Could you check a few things on this model? Use its own coordinates, in mm. A direction names the side the tool comes from. Round coordinates to 2 decimals unless told otherwise and drop trailing zeros. Order: outer loops, then holes, each group sorted by start corner. A loop starts at its lowest first (then second) coordinate and runs counter-clockwise, first axis right, second up.
```python
from build123d import *

# Parameters (mm, degrees)
EXTRUDE_1_DEPTH        = 60
HOLE_WIZARD_M6_1_D     = 5
HOLE_WIZARD_M6_1_DEPTH = 15
HOLE_WIZARD_M6_1_TIP   = 1.502151548
HOLE_WIZARD_M6_2_D     = 5
HOLE_WIZARD_M6_2_DEPTH = 15
HOLE_WIZARD_M6_2_TIP   = 1.502151548


with BuildPart() as part:
    # 草图1 → 凸台-拉伸1 (new body)
    with BuildSketch(Plane.XY):
        Polygon((0, 80), (0, 0), (80, 0), (80, 10), (10, 10), (10, 80), align=None)
    extrude(amount=EXTRUDE_1_DEPTH)

    # M6 螺纹孔1
    with Locations(Plane(origin=(65, 0, 50), x_dir=(0, 0, -1), z_dir=(0, -1, 0))):
        with Locations((0, 0), (40, 0), (40, -40), (0, -40)):
            Hole(HOLE_WIZARD_M6_1_D / 2, depth=HOLE_WIZARD_M6_1_DEPTH)
            with Locations((0, 0, -(HOLE_WIZARD_M6_1_DEPTH + HOLE_WIZARD_M6_1_TIP / 2))):  # 118° drill point
                Cone(0, HOLE_WIZARD_M6_1_D / 2, HOLE_WIZARD_M6_1_TIP, mode=Mode.SUBTRACT)

    # M6 螺纹孔2
    with Locations(Plane(origin=(0, 68, 9), x_dir=(0, 0, -1), z_dir=(-1, 0, 0))):
        with Locations((0, 0), (-42, 0)):
            Hole(HOLE_WIZARD_M6_2_D / 2, depth=HOLE_WIZARD_M6_2_DEPTH)
            with Locations((0, 0, -(HOLE_WIZARD_M6_2_DEPTH + HOLE_WIZARD_M6_2_TIP / 2))):  # 118° drill point
                Cone(0, HOLE_WIZARD_M6_2_D / 2, HOLE_WIZARD_M6_2_TIP, mode=Mode.SUBTRACT)


solid = part.part
```
Q1. For faces 5 (the flat face through (45, 10, 30)), 6 (the flat face through (22, 8, 0)), which set-ups out of +Z, -Z, +X, -X, +Y, -Y let a thin tool reach every point of the face, with its end or its side?
Q2. Imagine slicing it at D-D, the plane y = 31. Please give me the cut outline in (x, z), then the cut area to 3 significant figures.
Q3. Imagine slicing it at A-A, the plane x = 25. Please give me the cut outline in (y, z).
Q4. Imagine slicing it at B-B, the plane z = 50. Please give me the cut outline in (x, y), then the cut area to 3 significant figures.
Q5. For P1, Ø6, axis at x = 8, z = 42, coming from the -Y side; P2, Ø4, axis at x = 25, z = 50, coming from the +Y side; P3, Ø6, axis at x = 24.5, z = 7, coming from the +Y side; P4, Ø1, axis at y = 70.5, z = 36.5, coming from the +X side, each with a flat end and sliding along its axis, tell me the tip position at first contact or that it passes through.
Q6. Imagine slicing it at C-C, the plane z = 17.5. Please give me the cut outline in (x, y).
Q7. I need wall thicknesses on L1, parallel to X at y = 3, z = 50; L2, parallel to Z at x = 6.25, y = 68; L3, parallel to Y at x = 2, z = 9. Which ranges of each line are inside material? Lowest first, please.
Q8. We'd pull the mould along Z, two halves only. Please class faces 1 (the flat face through (22, 8, 60)), 2 (the cylindrical face through (5.07, 70.22, 10.15)), 3 (the flat face through (39, 0, 30)), 4 (the cylindrical face through (67.48, 5.07, 9.67)): released by +Z, released by -Z, zero draft, split by the parting line, or undercut.
Filled in:
1. face 5: +Z, -Z, +X, +Y
1. face 6: -Z, +X, -X, +Y, -Y
2. outline: (0, 0) - (10, 0) - (10, 60) - (0, 60) - close
2. area: 600 mm2
3. outline: (0, 0) - (10, 0) - (10, 7.5) - (0, 7.5) - close; (0, 12.5) - (10, 12.5) - (10, 47.5) - (0, 47.5) - close; (0, 52.5) - (10, 52.5) - (10, 60) - (0, 60) - close
4. outline: (0, 0) - (22.5, 0) - (22.5, 10) - (10, 10) - (10, 65.71) - (0, 65.71) - close; (0, 70.29) - (10, 70.29) - (10, 80) - (0, 80) - close; (27.5, 0) - (62.5, 0) - (62.5, 10) - (27.5, 10) - close; (67.5, 0) - (80, 0) - (80, 10) - (67.5, 10) - close
4. area: 1,350 mm2
5. P1: stops at y = 0
5. P2: passes through
5. P3: stops at y = 10
5. P4: stops at x = 10
6. outline: (0, 0) - (80, 0) - (80, 10) - (10, 10) - (10, 80) - (0, 80) - close
7. L1: x = 0 to 22.5, 27.5 to 62.5, 67.5 to 80
7. L2: z = 0 to 6.5, 11.5 to 48.5, 53.5 to 60
7. L3: y = 0 to 65.5, 70.5 to 80
8. face 1: released by +Z
8. face 2: undercut
8. face 3: zero draft
8. face 4: undercut
